```python
from build123d import *

# Parameters (mm, degrees)
SKETCH1_W                 = 281.36
SKETCH1_H                 = 30
BOSS_EXTRUDE1_DEPTH       = 3.18
CUT_EXTRUDE1_REACH        = 143.513
SKETCH2_R                 = 1.35
SKETCH2_R_2               = 1.425
MIRROR2_COPY_1_REACH      = 143.513
MIRROR2_COPY_1_SKETCH_R   = 1.35
MIRROR2_COPY_1_SKETCH_R_2 = 1.425
SKETCH3_W                 = 275
SKETCH3_H                 = 3.19
CUT_EXTRUDE2_DEPTH        = 3.18
SKETCH4_W                 = 3.18
SKETCH4_H                 = 281.36
BOSS_EXTRUDE2_DEPTH       = 12


with BuildPart() as part:
    # Sketch1 → Boss-Extrude1 (new body)
    with BuildSketch(Plane(origin=(0, 0, 0), x_dir=(0, 0, -1), z_dir=(1, 0, 0))):
        Rectangle(SKETCH1_W, SKETCH1_H)
    extrude(amount=BOSS_EXTRUDE1_DEPTH)

    # Sketch2 → Cut-Extrude1 (cut, up to next)
    with BuildSketch(Plane.ZY, mode=Mode.PRIVATE) as cut_extrude1_sk1:
        with Locations((-127.5, 10)):
            Circle(SKETCH2_R)
    cut_extrude1_tool1 = extrude(cut_extrude1_sk1.sketch, amount=-CUT_EXTRUDE1_REACH, mode=Mode.PRIVATE) & part.part
    # Sketch2 → Cut-Extrude1 (cut, up to next)
    with BuildSketch(Plane.ZY, mode=Mode.PRIVATE) as cut_extrude1_sk2:
        with Locations((-47.91, 10)):
            Circle(SKETCH2_R_2)
    cut_extrude1_tool2 = extrude(cut_extrude1_sk2.sketch, amount=-CUT_EXTRUDE1_REACH, mode=Mode.PRIVATE) & part.part
    cut_extrude1_1 = cut_extrude1_tool1.solids().sort_by_distance((0, 10, -127.5))[0]
    add(cut_extrude1_1, mode=Mode.SUBTRACT)
    cut_extrude1_2 = cut_extrude1_tool2.solids().sort_by_distance((0, 10, -47.91))[0]
    add(cut_extrude1_2, mode=Mode.SUBTRACT)
    cut_extrude1 = cut_extrude1_1 + cut_extrude1_2  # Cut-Extrude1 as one shape, for the pattern or mirror that repeats it

    # Mirror1: Cut-Extrude1 across plane
    add(cut_extrude1.mirror(Plane.ZX), mode=Mode.SUBTRACT)

    # Mirror2: Cut-Extrude1 across plane
    add(cut_extrude1.mirror(Plane.XY), mode=Mode.SUBTRACT)

    # Mirror2 copy 1 sketch → Mirror2 copy 1 (cut, up to next)
    with BuildSketch(Plane(origin=(0, 0, 0), x_dir=(0, 0, -1), z_dir=(-1, 0, 0)), mode=Mode.PRIVATE) as mirror2_copy_1_sk1:
        with Locations((-127.5, 10)):
            Circle(MIRROR2_COPY_1_SKETCH_R)
    mirror2_copy_1_tool1 = extrude(mirror2_copy_1_sk1.sketch, amount=-MIRROR2_COPY_1_REACH, mode=Mode.PRIVATE) & part.part
    # Mirror2 copy 1 sketch → Mirror2 copy 1 (cut, up to next)
    with BuildSketch(Plane(origin=(0, 0, 0), x_dir=(0, 0, -1), z_dir=(-1, 0, 0)), mode=Mode.PRIVATE) as mirror2_copy_1_sk2:
        with Locations((-47.91, 10)):
            Circle(MIRROR2_COPY_1_SKETCH_R_2)
    mirror2_copy_1_tool2 = extrude(mirror2_copy_1_sk2.sketch, amount=-MIRROR2_COPY_1_REACH, mode=Mode.PRIVATE) & part.part
    add(mirror2_copy_1_tool1.solids().sort_by_distance((0, -10, 127.5))[0], mode=Mode.SUBTRACT)
    add(mirror2_copy_1_tool2.solids().sort_by_distance((0, -10, 47.91))[0], mode=Mode.SUBTRACT)

    # Sketch3 → Cut-Extrude2 (cut)
    with BuildSketch(Plane(origin=(3.18, 0, 0), x_dir=(0, 0, -1), z_dir=(1, 0, 0))):
        with Locations((0, -1.615)):
            Rectangle(SKETCH3_W, SKETCH3_H)
    extrude(amount=-CUT_EXTRUDE2_DEPTH, mode=Mode.SUBTRACT)

    # Sketch4 → Boss-Extrude2 (add)
    with BuildSketch(Plane(origin=(0, 15, 0), x_dir=(1, 0, 0), z_dir=(0, 1, 0))):
        with Locations((1.59, 0)):
            Rectangle(SKETCH4_W, SKETCH4_H)
    extrude(amount=BOSS_EXTRUDE2_DEPTH)


solid = part.part
```
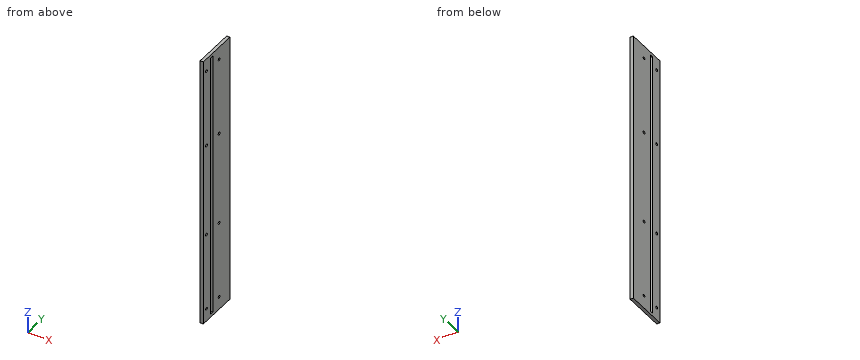
Geometry check sheet. Reference: the model listing, model coordinates, mm. Round coordinates to 2 decimals unless told otherwise and drop trailing zeros. Order: outer loops, then holes, each group sorted by start corner. A loop starts at its lowest first (then second) coordinate and runs counter-clockwise, first axis right, second up. Notation, with made-up numbers: (44.25, 30) - (48.25, 30) arc R34 cw to (48.25, 62) - close; hole circle Ø2 at (36, 70.5). An arc over 180 degrees is marked (long way). Use a Markdown table: item, result. Add a question column.
1) Section check B-B (x = 0.55). Count the separate pieces of the cut face and the enclosed holes in it, then the cut area to 3 significant figures.
2) Gauge pin test, flat end, axial feed: P1, Ø2.5, axis at y = -10, z = -47.91, coming from the +X side. Record the tip position at first contact, or that the pin passes through.
3) Thickness scan on line 1 along Y through (x, z) = (1.4, 47.91) (3 decimals); line 2 along Z through (x, y) = (1.8, -10) (3 decimals); line 3 along Y through (x, z) = (2, -127.5). Record the ranges inside material, lowest first.
4) Section check A-A (z = 90.5). Record the cut outline in (x, y), then the cut area to 3 significant figures.
Established:
| question | item | result |
|---|---|---|
| 1 | separate pieces | 1 |
| 1 | enclosed holes | 9 |
| 1 | area | 10,900 mm2 |
| 2 | P1 | through |
| 3 | line 1 | -15 to -11.425, -8.575 to -3.21, -0.02 to 8.575, 11.425 to 27 |
| 3 | line 2 | -140.68 to -128.85, -126.15 to -49.335, -46.485 to 46.485, 49.335 to 126.15, 128.85 to 140.68 |
| 3 | line 3 | -15 to -11.35, -8.65 to -3.21, -0.02 to 8.65, 11.35 to 27 |
| 4 | outline | (0, -15) - (3.18, -15) - (3.18, -3.21) - (0, -3.21) - close; (0, -0.02) - (3.18, -0.02) - (3.18, 27) - (0, 27) - close |
| 4 | area | 123 mm2 |
